For this review, take the finished solid that the model builds, in its own axes (mm). A direction names the side the tool comes from. Round coordinates to 2 decimals unless told otherwise and drop trailing zeros. Order: outer loops, then holes, each group sorted by start corner. A loop starts at its lowest first (then second) coordinate and runs counter-clockwise, first axis right, second up. Notation, with made-up numbers: (7.5, -24) - (21.5, -24) arc R12 ccw to (21.5, -5) - close; hole circle Ø7 at (-28, -10). An arc over 180 degrees is marked (long way). Write each question's results on one line, items separated by ' | '. Start each with the question number.
(1) Insertion check: pin 1 Ø4 at (x, z) = (-9, -0.5) entering from -Y; pin 2 Ø12.5 at (x, y) = (2.5, 0) entering from -Z; pin 3 Ø6.5 at (y, z) = (10.5, -5.5) entering from +X; pin 4 Ø12 at (y, z) = (-5, -13.5) entering from -X. Each pin has a flat end and moves straight along its axis. Give the tip position at first contact, or say it passes through.
(2) Draft analysis for pull direction X (two halves, no side actions). For faces 1 (the cylindrical face through (-19.006, 9.542, -12.214)), 2 (the flat face through (-13, 10, -6)), 3 (the cylindrical face through (-34.958, -0.275, 30.497)), state which applies: pulls with the +X half, pulls with the -X half, needs draft (parallel to the pull), parting line crosses it, or undercut.
(3) Take a section at D-D, the plane z = 1. Give the boundary of the cut face in (x, y).
(4) For L1, parallel to Z at x = -35.5, y = 0; L2, parallel to Y at x = -33, z = -10.5; L3, parallel to Z at x = -28, y = -10.75, list the stretches that pass through material, from the lowest coordinate up. Write a range as from..to.
(5) Take a section at C-C, the plane z = 15. Give the boundary of the cut face in (x, y).
(6) Take a section at A-A, the plane y = 0. Give the boundary of the cut face in (x, z), plus the area to 3 significant figures.
(7) For faces 4 (the flat face through (-8, 0, 6)), 5 (the cylindrical face through (-34.958, 0.846, 24.445)), 6 (the flat face through (32, -10, 3)), 7 (the flat face through (-31, 6.5, -7)), 8 (the flat face through (22, -6.5, 3)), list the 3-axis set-ups (+Z, -Z, +X, -X, +Y, -Y) from which the entire face can be reached by the end or side of a thin tool; tool diameter is ignored.
(8) Take a section at B-B, the plane x = -25.5. Give the boundary of the cut face in (y, z).
```python
from build123d import *

# Parameters (mm, degrees)
F1_DEPTH = 6
F2_R     = 6.5
F3_DEPTH = 6
F4_R     = 6.5
F5_DEPTH = 6


with BuildPart() as f1:
    # F0 (on Top) → F1 (new body)
    with BuildSketch(Plane.XY):
        with BuildLine():
            Line((-32, -12.5), (32, -12.5))
            Line((32, -12.5), (32, -6.5))
            Line((32, -6.5), (12, -6.5))
            ThreePointArc((12, -6.5), (5.5, 0), (12, 6.5))
            Line((12, 6.5), (32, 6.5))
            Line((32, 6.5), (32, 12.5))
            Line((32, 12.5), (-32, 12.5))
            Line((-32, 12.5), (-32, -12.5))
        make_face()
    extrude(amount=F1_DEPTH)

    # F2 (on face) → F3 (join)
    with BuildSketch(Plane(origin=(-32, 0, 0), x_dir=(0, -1, 0), z_dir=(-1, 0, 0))):
        with BuildLine():
            Line((-12.5, 18), (-12.5, 0))
            Line((-12.5, 0), (12.5, 0))
            Line((12.5, 0), (12.5, 18))
            ThreePointArc((12.5, 18), (0, 30.5), (-12.5, 18))
        make_face()
        with Locations((0, 18)):
            Circle(F2_R, mode=Mode.SUBTRACT)
    extrude(amount=F3_DEPTH)

    # F4 (on face) → F5 (join)
    with BuildSketch(Plane(origin=(0, 12.5, 0), x_dir=(-1, 0, 0), z_dir=(0, 1, 0))):
        with BuildLine():
            Line((38, -12.5), (38, 0))
            Line((38, 0), (13, 0))
            Line((13, 0), (13, -12.5))
            ThreePointArc((13, -12.5), (25.5, -25), (38, -12.5))
        make_face()
        with Locations((25.5, -12.5)):
            Circle(F4_R, mode=Mode.SUBTRACT)
    extrude(amount=-F5_DEPTH)


solid = f1.part
```
Results below:
1) pin 1: stops at y = -12.5 | pin 2: stops at z = 0 | pin 3: stops at x = -13 | pin 4: passes through
2) face 1: undercut | face 2: pulls with the +X half | face 3: needs draft
3) outline: (-38, -12.5) - (32, -12.5) - (32, -6.5) - (12, -6.5) arc R6.5 cw to (12, 6.5) - (32, 6.5) - (32, 12.5) - (-38, 12.5) - close
4) L1: z = 0..11.5, 24.5..30.5 | L2: y = 6.5..12.5 | L3: z = 0..6
5) outline: (-38, -12.5) - (-32, -12.5) - (-32, -5.77) - (-38, -5.77) - close; (-38, 5.77) - (-32, 5.77) - (-32, 12.5) - (-38, 12.5) - close
6) outline: (-38, 0) - (5.5, 0) - (5.5, 6) - (-32, 6) - (-32, 11.5) - (-38, 11.5) - close; (-38, 24.5) - (-32, 24.5) - (-32, 30.5) - (-38, 30.5) - close | area: 330 mm^2
7) face 4: +Z, +X, +Y, -Y | face 5: +X, -X | face 6: +Z, -Z, +X, +Y, -Y | face 7: -Z, +X, -X, -Y | face 8: +Z, -Z, +X
8) outline: (-12.5, 0) - (6.5, 0) - (6.5, -6) - (12.5, -6) - (12.5, 6) - (-12.5, 6) - close; (6.5, -25) - (12.5, -25) - (12.5, -19) - (6.5, -19) - close
